Here's how the part is built. I have some questions about the finished solid (model axes, mm). A direction names the side the tool comes from. Round coordinates to 2 decimals unless told otherwise and drop trailing zeros. Order: outer loops, then holes, each group sorted by start corner. A loop starts at its lowest first (then second) coordinate and runs counter-clockwise, first axis right, second up.
```python
from build123d import *

# Parameters (mm, degrees)
SKETCH3_R          = 2
CUT_EXTRUDE2_DEPTH = 0.5
SKETCH5_R          = 1.5
CUT_EXTRUDE3_DEPTH = 14.536986433
CHAMFER1_SIZE      = 0.1


with BuildPart() as part:
    # Sketch2 → Revolve1 (revolve)
    with BuildSketch(Plane.XY, mode=Mode.PRIVATE) as revolve1_sk:
        Polygon((0, 0), (0, 12), (1.5, 12), (1.5, 9.5), (3, 9.5), (3, 2.5), (1.5, 2.5), (1.5, 0), align=None)
    revolve(revolve1_sk.sketch.rotate(Axis((0, 0, 0), (0, 1, 0)), 90), axis=Axis((0, 0, 0), (0, 1, 0)))

    # Sketch3 → Cut-Extrude2 (cut)
    with BuildSketch(Plane.XY.offset(3)):
        with Locations((0, 6)):
            Circle(SKETCH3_R)
    cut_extrude2 = extrude(amount=-CUT_EXTRUDE2_DEPTH, mode=Mode.SUBTRACT)

    # Mirror1: Cut-Extrude2 across plane
    add(cut_extrude2.mirror(Plane.XY), mode=Mode.SUBTRACT)

    # Sketch5 → Cut-Extrude3 (cut, through all)
    with BuildSketch(Plane.XY.offset(2.5)):
        with Locations((0, 6)):
            Circle(SKETCH5_R)
    extrude(amount=-CUT_EXTRUDE3_DEPTH, mode=Mode.SUBTRACT)

    # Chamfer1
    chamfer1_edges = [part.edges().sort_by_distance(p)[0] for p in [
        (0, 0, 1.5),
        (0, 2.5, 3),
        (0, 9.5, 3),
        (0, 12, 1.5),
    ]]
    chamfer(chamfer1_edges, length=CHAMFER1_SIZE)


solid = part.part
```
1. If we section it at D-D, the plane y = 9: Write out the boundary of the cut face in (x, z), and give its area (3 significant figures).
Evaluation:
outline: circle Ø6 at (0, 0)
area: 28.3 mm2
2. If we mould it in two halves opening along X, with no side actions, what happens to faces 6 (the cylindrical face through (-0.45, 1.28, -1.43)), 7 (the cylindrical face through (0, 8, 2.7)), 8 (the flat face through (0, 0, 0))? For each: released by +X, released by -X, zero draft, split by the parting line, or undercut.
Evaluation:
face 6: split by the parting line
face 7: undercut
face 8: zero draft
3. If we section it at C-C, the plane z = 0: Write out the boundary of the cut face in (x, y).
Evaluation:
outline: (-3, 2.6) - (-2.9, 2.5) - (-1.5, 2.5) - (-1.5, 0.1) - (-1.4, 0) - (1.4, 0) - (1.5, 0.1) - (1.5, 2.5) - (2.9, 2.5) - (3, 2.6) - (3, 9.4) - (2.9, 9.5) - (1.5, 9.5) - (1.5, 11.9) - (1.4, 12) - (-1.4, 12) - (-1.5, 11.9) - (-1.5, 9.5) - (-2.9, 9.5) - (-3, 9.4) - close; hole circle Ø3 at (0, 6)
4. On a 3-axis mill with a long thin cutter (end or side, diameter ignored), from which of +Z, -Z, +X, -X, +Y, -Y can I reach the whole of each face in a straight line? I mean faces 1 (the cylindrical face through (0, 4, 2.7)), 2 (the flat face through (1.2, 9.5, 1.2)), 3 (the cylindrical face through (1.8, 6, 2.4)), 4 (the flat face through (1.2, 2.5, -1.2)), 5 (the cylindrical face through (0, 8, -2.7)). Say none if no direction works.
Evaluation:
face 1: +Z
face 2: +Y
face 3: +Y, -Y
face 4: -Y
face 5: -Z
5. I'm going to push flat-ended pins straight in: P1, Ø1, axis at x = -1, y = 5.5, coming from the +Z side; P2, Ø1, axis at y = 3, z = 2, coming from the -X side. Where does each tip first touch, or does it pass through?
Evaluation:
P1: stops at z = 2.5
P2: stops at x = -2.6
6. I need wall thicknesses on probe 1 along Y at (x, z) = (-1, -2); probe 2 along Y at (x, z) = (0, 0.9); probe 3 along X at (y, z) = (1.5, 0). Which ranges of each line are inside material? Lowest first, please.
Evaluation:
probe 1: y = 2.5 to 4.88, 7.12 to 9.5
probe 2: y = 0 to 4.5, 7.5 to 12
probe 3: x = -1.5 to 1.5
7. If we section it at A-A, the plane y = 6: Write out the boundary of the cut face in (x, z), and give its area (3 significant figures).
Evaluation:
outline: (-1.66, -2.5) - (-1.5, -2.5) - (-1.5, 2.5) - (-1.66, 2.5) arc R3 ccw to start; (1.5, -2.5) - (1.66, -2.5) arc R3 ccw to (1.66, 2.5) - (1.5, 2.5) - close
area: 11.0 mm2
